The model under review builds one solid part; all positions refer to its coordinate system, in mm. A direction names the side the tool comes from. Give positions to 0.01 mm unless a question says otherwise; leave off trailing zeros. Write each loop counter-clockwise with the first axis right and the second up, starting at its lowest first coordinate (ties: lowest second). Pieces come first, ordered by that corner, then holes.
from build123d import *

# Parameters (mm, degrees)
SKETCH2_R               = 16.2
BOSS_EXTRUDE2_DEPTH     = 10
SKETCH3_R               = 16.2
SKETCH3_R_2             = 1
CUT_EXTRUDE2_DEPTH      = 10
SKETCH4_R               = 16.2
SKETCH4_R_2             = 15
BOSS_EXTRUDE3_DEPTH     = 10
SKETCH7_R               = 1.375
CUT_EXTRUDE3_DEPTH      = 25
CUT_EXTRUDE3_DEPTH_BACK = 25
SKETCH8_R               = 1.375
CUT_EXTRUDE4_DEPTH      = 25
CUT_EXTRUDE4_DEPTH_BACK = 25


with BuildPart() as part:
    # Sketch2 → Boss-Extrude2 (new body)
    with BuildSketch(Plane(origin=(0, 0, 0), x_dir=(1, 0, 0), z_dir=(0, 1, 0))):
        with BuildLine():
            Line((33.90162956, 14.020502411), (7.113925389, 36.546463106))
            ThreePointArc((7.113925389, 36.546463106), (-3.831561071, 40.010315675), (-14.020502411, 34.720001617))
            Line((-14.020502411, 34.720001617), (-36.546463106, 7.932297446))
            ThreePointArc((-36.546463106, 7.932297446), (-40.010315675, -3.013189014), (-34.720001617, -13.202130354))
            Line((-34.720001617, -13.202130354), (-7.932297446, -35.728091049))
            ThreePointArc((-7.932297446, -35.728091049), (3.013189014, -39.191943618), (13.202130354, -33.90162956))
            Line((13.202130354, -33.90162956), (35.728091049, -7.113925389))
            ThreePointArc((35.728091049, -7.113925389), (39.191943618, 3.831561071), (33.90162956, 14.020502411))
        make_face()
        with Locations((-0.409186029, 0.409186029)):
            Circle(SKETCH2_R, mode=Mode.SUBTRACT)
    extrude(amount=BOSS_EXTRUDE2_DEPTH)

    # Sketch3 → Cut-Extrude2 (cut)
    with BuildSketch(Plane(origin=(0, 10, 0), x_dir=(1, 0, 0), z_dir=(0, 1, 0))):
        with Locations((-0.409186029, 0.409186029)):
            Circle(SKETCH3_R)
        with Locations((-34.010315675, -2.376211247)):
            Circle(SKETCH3_R_2)
        with Locations((-3.194583304, 34.010315675)):
            Circle(SKETCH3_R_2)
        with Locations((33.191943618, 3.194583304)):
            Circle(SKETCH3_R_2)
        with Locations((2.376211247, -33.191943618)):
            Circle(SKETCH3_R_2)
    extrude(amount=-CUT_EXTRUDE2_DEPTH, mode=Mode.SUBTRACT)

    # Sketch4 → Boss-Extrude3 (add)
    with BuildSketch(Plane(origin=(0, 10, 0), x_dir=(1, 0, 0), z_dir=(0, 1, 0))):
        with Locations((-0.409186029, 0.409186029)):
            Circle(SKETCH4_R)
        with Locations((-0.409186029, 0.409186029)):
            Circle(SKETCH4_R_2, mode=Mode.SUBTRACT)
    extrude(amount=-BOSS_EXTRUDE3_DEPTH)

    # Sketch7 → Cut-Extrude3 (cut, two sides)
    with BuildSketch(Plane(origin=(-0.371052455, 0, 0.032066779), x_dir=(-0.08610022, 0, -0.996286481), z_dir=(0.996286481, 0, -0.08610022))) as cut_extrude3_sk:
        with Locations((0.442897516, 5)):
            Circle(SKETCH7_R)
    extrude(amount=CUT_EXTRUDE3_DEPTH, mode=Mode.SUBTRACT)
    extrude(cut_extrude3_sk.sketch, amount=-CUT_EXTRUDE3_DEPTH_BACK, mode=Mode.SUBTRACT)

    # Sketch8 → Cut-Extrude4 (cut, two sides)
    with BuildSketch(Plane(origin=(-0.038133574, 0, -0.441252807), x_dir=(0.996286481, 0, -0.08610022), z_dir=(0.08610022, 0, 0.996286481))) as cut_extrude4_sk:
        with Locations((-0.372435501, 5)):
            Circle(SKETCH8_R)
    extrude(amount=CUT_EXTRUDE4_DEPTH, mode=Mode.SUBTRACT)
    extrude(cut_extrude4_sk.sketch, amount=-CUT_EXTRUDE4_DEPTH_BACK, mode=Mode.SUBTRACT)


solid = part.part
1) Consider section A-A, the plane z = -6. Give the boundary of the cut face in (x, y).
2) Consider section B-B, the plane x = -13. Give the boundary of the cut face in (y, z).
3) To check wall thickness, follow probe 1 along X at (y, z) = (4.5, 19); probe 2 along Z at (x, y) = (9, 4.25); probe 3 along Z at (x, y) = (-2, 6.75). State the ranges of each line that lie inside material, in increasing order.
4) Consider section C-C, the plane y = 7.75. Give the boundary of the cut face in (x, z), then the cut area to 3 significant figures.
5) Insertion check: pin 1 (6 mm diameter, centred on y = 2, z = -21.5, fed in from +X); pin 2 (6 mm diameter, centred on y = 8.5, z = -15.5, fed in from +X); pin 3 (1 mm diameter, centred on y = 2, z = 24.5, fed in from -X). Each pin has a flat end and moves straight along its axis. Give the tip position at first contact, or say it passes through.
6) The part is to be moulded in two halves that separate along Z. For faces 3 (the flat face through (17, 10, -1)), 4 (the cylindrical face through (2.849, 4.93, 39.205)), 5 (the cylindrical face through (-2.301, 6.363, -20.217)), say which applies: +Z half, -Z half, draft (parallel to the pull), parting line (faces both ways), or undercut.
7) Tool access review of faces 1 (the flat face through (-21.51, 4.93, 24.31)), 2 (the flat face through (24.5, 5.02, -2.54)): name each direction out of +Z, -Z, +X, -X, +Y, -Y from which nothing blocks a thin tool from reaching the whole face with its end or side.
8) Consider section D-D, the plane z = 28. Give the boundary of the cut face in (x, y).
Answer block:
1. outline: (-37.93, 0) - (-14.33, 0) - (-14.33, 10) - (-37.93, 10) - close; (13.51, 0) - (38.84, 0) - (38.84, 10) - (13.51, 10) - close
2. outline: (0, -35.82) - (10, -35.82) - (10, -8.56) - (0, -8.56) - close; (0, 7.74) - (10, 7.74) - (10, 31.47) - (0, 31.47) - close
3. probe 1: x = -27.83 to -0.02, 2.55 to 25.73
3. probe 2: z = -34.96 to -12.09, 11.27 to 37.36
3. probe 3: z = -40.06 to -15.32, 14.51 to 38.78
4. outline: (-36.55, -7.93) - (-14.02, -34.72) arc R15 ccw to (7.11, -36.55) - (33.9, -14.02) arc R15 ccw to (35.73, 7.11) - (13.2, 33.9) arc R15 ccw to (-7.93, 35.73) - (-34.72, 13.2) arc R15 ccw to start; hole circle Ø2 at (-34.01, 2.38); hole circle Ø30 at (-0.41, -0.41); hole circle Ø2 at (-3.19, -34.01); hole circle Ø2 at (2.38, 33.19); hole circle Ø2 at (33.19, -3.19)
4. area: 3,310 mm2
5. pin 1: stops at x = 28.57
5. pin 2: stops at x = 35.46
5. pin 3: stops at x = -21.88
6. face 3: draft
6. face 4: +Z half
6. face 5: undercut
7. face 1: +Z, -X, +Y, -Y
7. face 2: none
8. outline: (-17.12, 0) - (18.16, 0) - (18.16, 10) - (-17.12, 10) - close
